```python
from build123d import *

# Parameters (mm, degrees)
SKETCH1_W                                  = 120
SKETCH1_H                                  = 50
BASE_FLANGE1_DEPTH                         = 5
EDGE_FLANGE1_STRIP_W                       = 30
EDGE_FLANGE1_STRIP_H                       = 5
EDGE_FLANGE1_STRIP_CUT_DEPTH               = 120
EDGE_FLANGE1_DEPTH                         = 120
CUT_EXTRUDE1_DEPTH                         = 10
CBORE_FOR_M3_CHEESE_HEAD_SCREW1_AT_2_COUNT = 2
CBORE_FOR_M3_CHEESE_HEAD_SCREW1_AT_2_PITCH = 47.5
CBORE_FOR_M3_CHEESE_HEAD_SCREW1_AT_3_COUNT = 2
CBORE_FOR_M3_CHEESE_HEAD_SCREW1_AT_3_PITCH = 95
BREAK_CORNER1_START                        = -30
BREAK_CORNER1_DEPTH                        = 5
BREAK_CORNER1_2_DEPTH                      = 5


# Read off the part's stored shape, not the designer's step: Break-Corner1
# Sheet-metal steps are written as plain solids
with BuildPart() as part:
    # Sketch1 → Base-Flange1 (new body)
    with BuildSketch(Plane(origin=(0, 0, 0), x_dir=(1, 0, 0), z_dir=(0, 1, 0))):
        Rectangle(SKETCH1_W, SKETCH1_H)
    extrude(amount=BASE_FLANGE1_DEPTH)

    # Edge-Flange1 strip (across the edge) → Edge-Flange1 strip cut (cut)
    with BuildSketch(Plane(origin=(60, 5, -25), x_dir=(0, 0, 1), z_dir=(-1, 0, 0))):
        with Locations((-10, -2.5)):
            Rectangle(EDGE_FLANGE1_STRIP_W, EDGE_FLANGE1_STRIP_H)
    extrude(amount=EDGE_FLANGE1_STRIP_CUT_DEPTH, mode=Mode.SUBTRACT)

    # Edge-Flange1 section (across the edge) → Edge-Flange1 (add)
    with BuildSketch(Plane(origin=(60, 5, -25), x_dir=(0, 0, 1), z_dir=(-1, 0, 0))):
        with BuildLine():
            Line((-5, 5), (-5, 15))
            Line((-5, 15), (0, 15))
            Line((0, 15), (0, 5))
            ThreePointArc((0, 5), (1.464466094, 1.464466094), (5, 0))
            Line((5, 0), (5, -5))
            ThreePointArc((5, -5), (-2.071067812, -2.071067812), (-5, 5))
        make_face()
    extrude(amount=EDGE_FLANGE1_DEPTH)

    # Sketch9 → Cut-Extrude1 (cut)
    with BuildSketch(Plane(origin=(0, 5, 0), x_dir=(1, 0, 0), z_dir=(0, 1, 0))):
        with BuildLine():
            Line((-10, -25), (-10, -16.613247726))
            ThreePointArc((-10, -16.613247726), (-10.594600569, -13.216416623), (-12.307692308, -10.223537062))
            ThreePointArc((-12.307692308, -10.223537062), (0, 16), (12.307692308, -10.223537062))
            ThreePointArc((12.307692308, -10.223537062), (10.594600569, -13.216416623), (10, -16.613247726))
            Line((10, -16.613247726), (10, -25))
            Line((10, -25), (-10, -25))
        make_face()
    extrude(amount=-CUT_EXTRUDE1_DEPTH, mode=Mode.SUBTRACT)

    # Sketch14 → CBORE for M3 Cheese Head Screw1 (revolve, cut)
    with BuildSketch(Plane(origin=(-47.5, 15, -25), x_dir=(0, -1, 0), z_dir=(1, 0, 0))):
        Polygon((0, 0), (0, 5), (1.7, 5), (1.7, 2), (3.25, 2), (3.25, 0.025), (3.275, 0), align=None)
    cbore_for_m3_cheese_head_screw1 = revolve(axis=Axis((-47.5, 15, -18.65), (0, 0, -1)), mode=Mode.SUBTRACT)

    # CBORE for M3 Cheese Head Screw1 at 2: CBORE for M3 Cheese Head Screw1 ×2
    with Locations(*[(i * CBORE_FOR_M3_CHEESE_HEAD_SCREW1_AT_2_PITCH, 0, 0) for i in range(1, CBORE_FOR_M3_CHEESE_HEAD_SCREW1_AT_2_COUNT)]):
        add(cbore_for_m3_cheese_head_screw1, mode=Mode.SUBTRACT)

    # CBORE for M3 Cheese Head Screw1 at 3: CBORE for M3 Cheese Head Screw1 ×2
    with Locations(*[(i * CBORE_FOR_M3_CHEESE_HEAD_SCREW1_AT_3_PITCH, 0, 0) for i in range(1, CBORE_FOR_M3_CHEESE_HEAD_SCREW1_AT_3_COUNT)]):
        add(cbore_for_m3_cheese_head_screw1, mode=Mode.SUBTRACT)

    # Break-Corner1 outline → Break-Corner1 (cut)
    with BuildSketch(Plane.XY.offset(BREAK_CORNER1_START)):
        with BuildLine():
            Line((60, 20), (55, 20))
            ThreePointArc((55, 20), (58.535533906, 18.535533906), (60, 15))
            Line((60, 15), (60, 20))
        make_face()
        with BuildLine():
            ThreePointArc((-60, 15), (-58.535533906, 18.535533906), (-55, 20))
            Line((-55, 20), (-60, 20))
            Line((-60, 20), (-60, 15))
        make_face()
    extrude(amount=BREAK_CORNER1_DEPTH, mode=Mode.SUBTRACT)

    # Break-Corner1 2 outline → Break-Corner1 2 (cut)
    with BuildSketch(Plane(origin=(0, 0, 0), x_dir=(1, 0, 0), z_dir=(0, 1, 0))):
        with BuildLine():
            Line((60, -25), (60, -20))
            ThreePointArc((60, -20), (58.535533906, -23.535533906), (55, -25))
            Line((55, -25), (60, -25))
        make_face()
        with BuildLine():
            Line((-60, -25), (-55, -25))
            ThreePointArc((-55, -25), (-58.535533906, -23.535533906), (-60, -20))
            Line((-60, -20), (-60, -25))
        make_face()
    extrude(amount=BREAK_CORNER1_2_DEPTH, mode=Mode.SUBTRACT)


solid = part.part
```
Can you work these out from the model? Positions are in its coordinate system, mm. A direction names the side the tool comes from. Round coordinates to 2 decimals unless told otherwise and drop trailing zeros. Order: outer loops, then holes, each group sorted by start corner. A loop starts at its lowest first (then second) coordinate and runs counter-clockwise, first axis right, second up. Notation, with made-up numbers: (17, -5.5) -> (26, -5.5) arc R20 ccw to (26, 1.5) -> close; hole circle Ø5 at (68, 39). An arc over 180 degrees is marked (long way). Return JSON: item names as keys, results as strings. Group by question number.
1. I need wall thicknesses on line 1 (X direction, y = 15, z = -29.25); line 2 (X direction, y = 15, z = -25.65); line 3 (X direction, y = 2.8, z = 0). Which ranges of each line are inside material? Lowest first, please. Write a range as [from, to].
2. Will these pins go through, and if not, where does the flat tip stop? pin 1 (11 mm diameter, centred on x = 16.5, y = 17.5, fed in from +Z); pin 2 (13.5 mm diameter, centred on x = -14, z = -2.5, fed in from +Y); pin 3 (8 mm diameter, centred on x = -12, z = -20.5, fed in from +Y).
3. If we section it at B-B, the plane z = 0: Write out the boundary of the cut face in (x, y).
4. Which directions (+Z, -Z, +X, -X, +Y, -Y) give clear straight access to the entire face, cutting with the end or side of a thin tool? Please do faces 4 (the face through (59, 2, 23)), 5 (the face through (0.8, 18.4, -25)), 6 (the face through (-10, 3, 21)), 7 (the face through (50.673, 15.705, -25.999)).
5. If we section it at A-A, the plane x = 0: Write out the boundary of the cut face in (y, z) (3 decimals).
6. If we section it at C-C, the plane x = 31: Write out the boundary of the cut face in (y, z), then the cut area to 3 significant figures.
7. We'd pull the mould along Z, two halves only. Please class faces 1 (the face through (1, 20, -28)), 2 (the face through (-33, 2, 25)), 3 (the face through (-10.58, 2.54, 13.26)): released by +Z, released by -Z, zero draft, split by the parting line, or undercut.
8. If we section it at D-D, the plane x = -47.5: Write out the boundary of the cut face in (y, z) (3 decimals).
Output values:
{
 "1": {"line 1": "[-60, -49.2], [-45.8, -1.7], [1.7, 45.8], [49.2, 60]", "line 2": "[-60, -50.75], [-44.25, -3.25], [3.25, 44.25], [50.75, 60]", "line 3": "[-60, -16], [16, 60]"},
 "2": {"pin 1": "z = -25", "pin 2": "y = 5", "pin 3": "y = 7.82"},
 "3": {"outline": "(-60, 0) -> (-16, 0) -> (-16, 5) -> (-60, 5) -> close; (16, 0) -> (60, 0) -> (60, 5) -> (16, 5) -> close"},
 "4": {"face 4": "+Z, +X, +Y, -Y", "face 5": "+Z, +X, -X, +Y", "face 6": "+Z, +Y, -Y", "face 7": "+Z"},
 "5": {"outline": "(0, -20) arc R10 ccw to (10, -30) -> (13.3, -30) -> (13.3, -27) -> (11.75, -27) -> (11.75, -25.025) -> (11.725, -25) -> (10, -25) arc R5 cw to (5, -20) -> (5, -16) -> (0, -16) -> close; (16.7, -30) -> (20, -30) -> (20, -25) -> (18.275, -25) -> (18.25, -25.025) -> (18.25, -27) -> (16.7, -27) -> close"},
 "6": {"outline": "(0, -20) arc R10 ccw to (10, -30) -> (20, -30) -> (20, -25) -> (10, -25) arc R5 cw to (5, -20) -> (5, 25) -> (0, 25) -> close", "area": "334 mm²"},
 "7": {"face 1": "zero draft", "face 2": "released by +Z", "face 3": "undercut"},
 "8": {"outline": "(0, -20) arc R10 ccw to (10, -30) -> (13.3, -30) -> (13.3, -27) -> (11.75, -27) -> (11.75, -25.025) -> (11.725, -25) -> (10, -25) arc R5 cw to (5, -20) -> (5, 25) -> (0, 25) -> close; (16.7, -30) -> (20, -30) -> (20, -25) -> (18.275, -25) -> (18.25, -25.025) -> (18.25, -27) -> (16.7, -27) -> close"}
}
